Design review of the part built by this model. Coordinates are the model's own, in mm. A direction names the side the tool comes from. Coordinates: 2 decimals unless noted, no trailing zeros. Order: outer loops, then holes, each group sorted by start corner. A loop starts at its lowest first (then second) coordinate and runs counter-clockwise, first axis right, second up. Notation, with made-up numbers: M 65,37.25 L 122,37.25 A19 cw 122,48.25 Z; hole C -1.75,6 d3. An arc over 180 degrees is marked long. Use CSV: the item, a comma, the result in double quotes.
```python
from build123d import *

# Parameters (mm, degrees)
SKETCH2_W                  = 5
SKETCH2_H                  = 8
BOSS_EXTRUDE1_DEPTH        = 25
M2_5_CLEARANCE_HOLE1_D     = 3
M2_5_CLEARANCE_HOLE1_DEPTH = 9.098709071
M2_5_CLEARANCE_HOLE1_TIP   = 0.901290929
SKETCH5_W                  = 2.5
SKETCH5_H                  = 5.1
CUT_EXTRUDE1_DEPTH         = 7.2
M2_5_CLEARANCE_HOLE2_D     = 3.1
SKETCH7_2_R                = 0.5
CUT_EXTRUDE2_DEPTH         = 2.5


with BuildPart() as part:
    # Sketch1 → Revolve1 (revolve)
    with BuildSketch(Plane(origin=(0, 0, 0), x_dir=(1, 0, 0), z_dir=(0, 1, 0)), mode=Mode.PRIVATE) as revolve1_sk:
        Polygon((0, 4), (-5, 4), (-9.525, 4), (-9.525, -16), (-5, -16), (-5, -27), (-3, -27), (-3, 0), (0, 0), align=None)
    revolve(revolve1_sk.sketch.rotate(Axis((0, 0, 0), (0, 0, -1)), 180), axis=Axis((0, 0, 0), (0, 0, -1)))

    # Sketch2 → Boss-Extrude1 (add)
    with BuildSketch(Plane(origin=(0, 0, -4), x_dir=(-1, 0, 0), z_dir=(0, 0, -1))):
        Rectangle(SKETCH2_W, SKETCH2_H)
    extrude(amount=BOSS_EXTRUDE1_DEPTH)

    # M2.5 Clearance Hole1
    with Locations(Plane(origin=(2.5, 0, 0), x_dir=(0, 0, -1), z_dir=(1, 0, 0))):
        with Locations((24, 0), (14, 0)):
            Hole(M2_5_CLEARANCE_HOLE1_D / 2, depth=M2_5_CLEARANCE_HOLE1_DEPTH)
            with Locations((0, 0, -(M2_5_CLEARANCE_HOLE1_DEPTH + M2_5_CLEARANCE_HOLE1_TIP / 2))):  # 118° drill point
                Cone(0, M2_5_CLEARANCE_HOLE1_D / 2, M2_5_CLEARANCE_HOLE1_TIP, mode=Mode.SUBTRACT)

    # Sketch5 → Cut-Extrude1 (cut)
    with BuildSketch(Plane.XZ.offset(4)):
        with Locations((0, -14)):
            Rectangle(SKETCH5_W, SKETCH5_H)
        with Locations((0, -24)):
            Rectangle(SKETCH5_W, SKETCH5_H)
    extrude(amount=-CUT_EXTRUDE1_DEPTH, mode=Mode.SUBTRACT)

    # M2.5 Clearance Hole2 (through all)
    with Locations(Plane.ZY.offset(9.525)):
        with Locations((7, 0)):
            Hole(M2_5_CLEARANCE_HOLE2_D / 2)

    # Sketch7<2> → Cut-Extrude2 (cut)
    with BuildSketch(Plane.ZY.offset(9.525)):
        Polygon((7, -2.944486373), (9.55, -1.472243186), (9.55, 1.472243186), (7, 2.944486373), (4.45, 1.472243186), (4.45, -1.472243186), align=None)
        with Locations((7, 0)):
            Circle(SKETCH7_2_R, mode=Mode.SUBTRACT)
    extrude(amount=-CUT_EXTRUDE2_DEPTH, mode=Mode.SUBTRACT)


solid = part.part
```
(1) Add section C-C on y = 0. Give the number of separate pieces and of enclosed holes in the cut face, and give its area (3 significant figures).
The answers:
separate pieces,"5"
enclosed holes,"0"
area,"368 mm2"
(2) Wall thickness on probe 1 along Z at (x, y) = (-5.1, 0); probe 2 along Y at (x, z) = (2, -24); probe 3 along X at (y, z) = (0.25, 17): over which ranges is each line inside the solid? List them lowest first.
The answers:
probe 1,"z = -4 to 5.45, 8.55 to 16"
probe 2,"y = -4 to -1.5, 1.5 to 4"
probe 3,"x = -4.99 to -2.99, 2.99 to 4.99"
(3) Add section A-A on z = -24. State the section outline as (x, y) points.
The answers:
outline,"M -2.5,-4 L -1.25,-4 L -1.25,-1.5 L -2.5,-1.5 Z; M -2.5,1.5 L -1.25,1.5 L -1.25,3.2 L 1.25,3.2 L 1.25,1.5 L 2.5,1.5 L 2.5,4 L -2.5,4 Z; M 1.25,-4 L 2.5,-4 L 2.5,-1.5 L 1.25,-1.5 Z"
(4) Add section D-D on z = 24. State the section outline as (x, y) points.
The answers:
outline,"C 0,0 d10; hole C 0,0 d6"
(5) Add section B-B on x = 0. State the section outline as (y, z) points (3 decimals), and give its area (3 significant figures).
The answers:
outline,"M -9.525,-4 L -4,-4 L -4,-11.45 L 3.2,-11.45 L 3.2,-16.55 L -4,-16.55 L -4,-21.45 L 3.2,-21.45 L 3.2,-26.55 L -4,-26.55 L -4,-29 L 4,-29 L 4,-4 L 9.525,-4 L 9.525,16 L 5,16 L 5,27 L 3,27 L 3,0 L -3,0 L -3,27 L -5,27 L -5,16 L -9.525,16 Z"
area,"456 mm2"
(6) Clearance check with flat-ended pins moving along their axes: P1, Ø0.8, axis at x = -7.5, y = 0.5, coming from the -Z side; P2, Ø5, axis at x = -3, z = 11, coming from the -Y side; P3, Ø2, axis at x = 3.5, z = 12, coming from the -Y side. State where each tip first meets the part, or that it passes through.
The answers:
P1,"stops at z = -4"
P2,"stops at y = -9.51"
P3,"stops at y = -9.19"
(7) The part is to be moulded in two halves that separate along Z. For faces 5 (the face through (2.5, 0, -16)), 6 (the face through (1.87, 0.07, -15.5)), 7 (the face through (-4, 0, -4)), say which applies: pulls with the +Z half, pulls with the -Z half, needs draft (parallel to the pull), parting line crosses it, or undercut.
The answers:
face 5,"needs draft"
face 6,"undercut"
face 7,"pulls with the -Z half"
(8) For faces 1 (the face through (-2.5, 0, -16)), 2 (the face through (2, -4, -16)), 3 (the face through (-8, 0, 4.45)), 4 (the face through (-1.25, -1.3, -25.2)), list the 3-axis set-ups (+Z, -Z, +X, -X, +Y, -Y) from which the entire face can be reached by the end or side of a thin tool; tool diameter is ignored.
The answers:
face 1,"-Z, -X, +Y, -Y"
face 2,"-Z, +X, -X, -Y"
face 3,"-X"
face 4,"-Y"
